Job drawing, mm, ordinate dimensions from the low corner. One solid piece. Coordinates: 2 decimals unless noted, no trailing zeros. Loops run counter-clockwise (first coordinate to the right, second up) from the corner with the lowest first, then second, coordinate; pieces in that order, holes last. Notation, with made-up numbers: M 71.5,68 L 129.5,68 A20 ccw 129.5,100 Z; hole C 17.25,51 d1. An arc over 180 degrees is marked long. Answer as a JSON object with one key per item and string values. Group by question number.
1. Drill centre lines: L1, parallel to Z at x = 24, y = 1.9; L2, parallel to X at y = 1.3, z = 6.5; L3, parallel to Z at x = 23, y = 0.6. Where is each one in solid material? Low to high.
2. Saw through at C-C on x = 19.5. Write the cut outline in (y, z), then the cut area to 3 significant figures.
3. Drop flat-ended pins along their axis: pin 1 Ø1.5 at (x, y) = (8.5, 1.5) entering from -Z; pin 2 Ø0.9 at (y, z) = (2, 49.5) entering from -X; pin 3 Ø0.9 at (y, z) = (2, 1.5) entering from -X. Give the stop position or say it passes through.
4. Saw through at B-B on x = 24. Write the cut outline in (y, z).
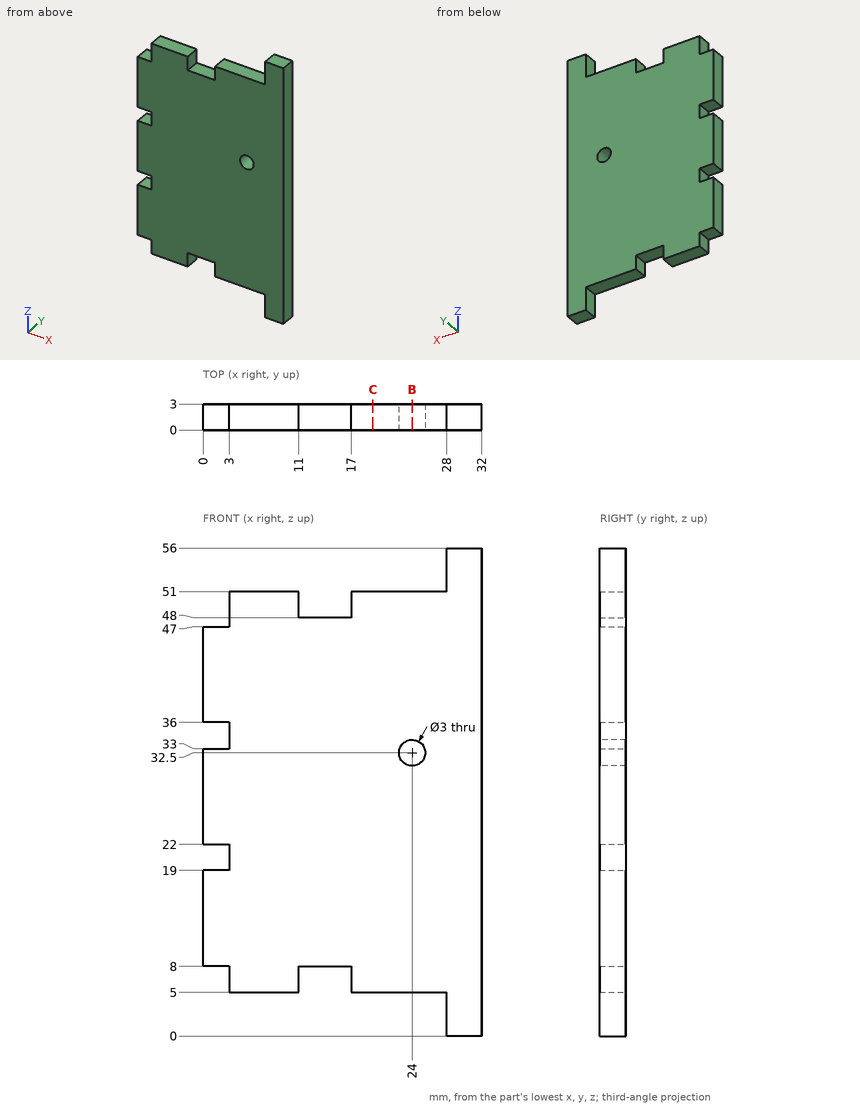
Outcome:
{
 "1": {"L1": "z = 5 to 31, 34 to 51", "L2": "x = 3 to 11, 17 to 32", "L3": "z = 5 to 31.38, 33.62 to 51"},
 "2": {"outline": "M 0,5 L 3,5 L 3,51 L 0,51 Z", "area": "138 mm²"},
 "3": {"pin 1": "stops at z = 5", "pin 2": "stops at x = 3", "pin 3": "stops at x = 28"},
 "4": {"outline": "M 0,5 L 3,5 L 3,31 L 0,31 Z; M 0,34 L 3,34 L 3,51 L 0,51 Z"}
}
